Can you work these out from the model? Positions are in its coordinate system, mm. A direction names the side the tool comes from. Give positions to 0.01 mm unless a question says otherwise; leave off trailing zeros. Loops run counter-clockwise (first coordinate to the right, second up) from the corner with the lowest first, then second, coordinate; pieces in that order, holes last.
from build123d import *

# Parameters (mm, degrees)
SKETCH1_W                        = 40
SKETCH1_H                        = 40
BOSS_EXTRUDE1_DEPTH              = 40
SKETCH2_R                        = 5
CUT_EXTRUDE1_DEPTH               = 61
FILLET1_R                        = 10
M6_5_CLEARANCE_HOLE1_D           = 7.1
M6_5_CLEARANCE_HOLE1_DEPTH       = 10
M6_5_CLEARANCE_HOLE1_CSINK_D     = 7.15
M6_5_CLEARANCE_HOLE1_CSINK_ANGLE = 100
M6_5_CLEARANCE_HOLE1_TIP         = 2.133055198
SKETCH6_R                        = 5
CUT_EXTRUDE2_DEPTH               = 10


with BuildPart() as part:
    # Sketch1 → Boss-Extrude1 (new body)
    with BuildSketch(Plane(origin=(0, 0, 0), x_dir=(1, 0, 0), z_dir=(0, 1, 0))):
        Rectangle(SKETCH1_W, SKETCH1_H)
    extrude(amount=BOSS_EXTRUDE1_DEPTH)

    # Sketch2 → Cut-Extrude1 (cut, through all)
    with BuildSketch(Plane.XY.offset(20)):
        with Locations((0, 20)):
            Circle(SKETCH2_R)
    extrude(amount=-CUT_EXTRUDE1_DEPTH, mode=Mode.SUBTRACT)

    # Fillet1
    fillet1_edges = [part.edges().sort_by_distance(p)[0] for p in [
        (-20, 40, 0),
        (20, 40, 0),
    ]]
    fillet(fillet1_edges, radius=FILLET1_R)

    # M6.5 Clearance Hole1
    with Locations(Plane(origin=(0, 0, 0), x_dir=(-1, 0, 0), z_dir=(0, -1, 0))):
        with Locations((-10, 10), (10, 10), (-10, -10), (10, -10)):
            CounterSinkHole(M6_5_CLEARANCE_HOLE1_D / 2, M6_5_CLEARANCE_HOLE1_CSINK_D / 2, depth=M6_5_CLEARANCE_HOLE1_DEPTH, counter_sink_angle=M6_5_CLEARANCE_HOLE1_CSINK_ANGLE)
            with Locations((0, 0, -(M6_5_CLEARANCE_HOLE1_DEPTH + M6_5_CLEARANCE_HOLE1_TIP / 2))):  # 118° drill point
                Cone(0, M6_5_CLEARANCE_HOLE1_D / 2, M6_5_CLEARANCE_HOLE1_TIP, mode=Mode.SUBTRACT)

    # Sketch6 → Cut-Extrude2 (cut)
    with BuildSketch(Plane.XZ):
        with Locations(Location((0, 0, 0), (0, 0, 270))):
            Circle(SKETCH6_R)
    extrude(amount=-CUT_EXTRUDE2_DEPTH, mode=Mode.SUBTRACT)


solid = part.part
(1) Please list where these lines run through material, in increasing order: probe 1 along Z at (x, y) = (-10, 3); probe 2 along Y at (x, z) = (0, -3); probe 3 along Y at (x, z) = (0, 7.5).
Returned:
probe 1: z = -20 to -13.55, -6.45 to 6.45, 13.55 to 20
probe 2: y = 10 to 15, 25 to 40
probe 3: y = 0 to 15, 25 to 40
(2) Suppose I cut it at A-A on x = 0. List the corners of the cut face in (y, z) for me.
Returned:
outline: (0, -20) - (15, -20) - (15, 20) - (0, 20) - (0, 5) - (10, 5) - (10, -5) - (0, -5) - close; (25, -20) - (40, -20) - (40, 20) - (25, 20) - close
(3) Will these pins go through, and if not, where does the flat tip stop? P1, Ø9, axis at x = 0, y = 20, coming from the +Z side; P2, Ø3, axis at x = -0.5, z = 1, coming from the -Y side; P3, Ø4, axis at x = 15, z = 15, coming from the +Y side; P4, Ø3, axis at x = -14, z = -5.5, coming from the +Y side.
Returned:
P1: passes through
P2: stops at y = 10
P3: stops at y = 39.54
P4: stops at y = 39.68
(4) Suppose I cut it at C-C on y = 19. List the corners of the cut face in (x, z) for me.
Returned:
outline: (-20, -20) - (-4.9, -20) - (-4.9, 20) - (-20, 20) - close; (4.9, -20) - (20, -20) - (20, 20) - (4.9, 20) - close
(5) Suppose I cut it at B-B on z = 0. List the corners of the cut face in (x, y) for me, plus the area to 3 significant figures.
Returned:
outline: (-20, 0) - (-5, 0) - (-5, 10) - (5, 10) - (5, 0) - (20, 0) - (20, 30) arc R10 ccw to (10, 40) - (-10, 40) arc R10 ccw to (-20, 30) - close; hole circle Ø10 at (0, 20)
area: 1,380 mm2
(6) Thinking about a two-plate mould opening in X: for faces 1 (the flat face through (-5, 0, -5)), 2 (the cylindrical face through (16.99, 37.15, -0.28)), 3 (the flat face through (-20, 15, 0)), 4 (the cylindrical face through (11.64, 5.08, -6.85)), which applies, pulls with the +X half, pulls with the -X half, needs draft (parallel to the pull), parting line crosses it, or undercut?
Returned:
face 1: needs draft
face 2: pulls with the +X half
face 3: pulls with the -X half
face 4: undercut
(7) Which directions (+Z, -Z, +X, -X, +Y, -Y) give clear straight access to the entire face, cutting with the end or side of a thin tool? Please do faces 5 (the cylindrical face through (-1.08, 15.12, 0.28)), 6 (the cylindrical face through (-4.88, 4.93, 1.08)).
Returned:
face 5: +Z, -Z
face 6: -Y
(8) Suppose I cut it at D-D on x = 16. List the corners of the cut face in (y, z) for me, plus the area to 3 significant figures.
Returned:
outline: (0, -20) - (38, -20) - (38, 20) - (0, 20) - close
area: 1,520 mm2
